Could you check a few things on this drawing? It's one solid part, dimensions in mm from its lowest x, y, z. Coordinates: 2 decimals unless noted, no trailing zeros. Write each loop counter-clockwise with the first axis right and the second up, starting at its lowest first coordinate (ties: lowest second). Pieces come first, ordered by that corner, then holes. Notation, with made-up numbers: M 13.5,-17 L 48.5,-17 A14 cw 48.5,2 Z; hole C 25.25,75 d1. An arc over 180 degrees is marked long. Use a Markdown table: item, result.
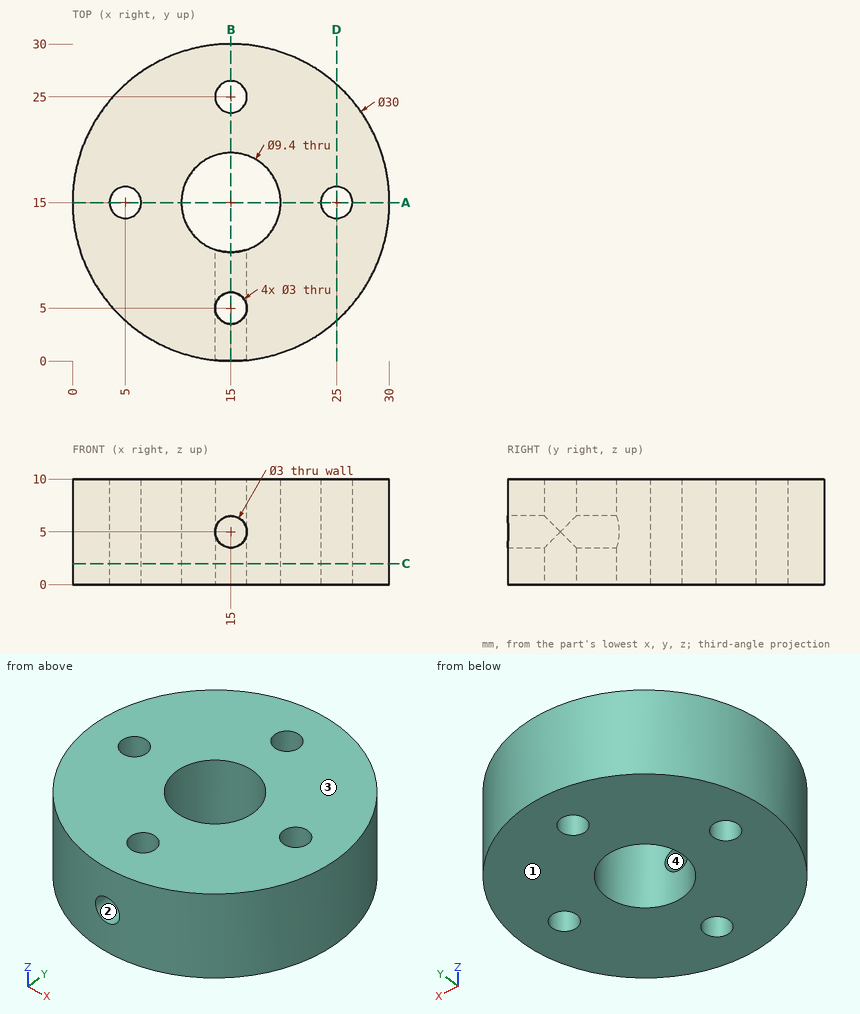
1. Suppose I cut it at C-C on z = 2. Write out the boundary of the cut face in (x, y), and give its area (3 significant figures).
Answers follow:
| item | result |
|---|---|
| outline | C 15,15 d30; hole C 5,15 d3; hole C 15,15 d9.4; hole C 15,5 d3; hole C 15,25 d3; hole C 25,15 d3 |
| area | 609 mm2 |
2. We'd pull the mould along Z, two halves only. Please class the marked faces 1, 2, 3 and 4: +Z half, -Z half, draft (parallel to the pull), parting line (faces both ways), or undercut.
Answers follow:
| item | result |
|---|---|
| face 1 | -Z half |
| face 2 | undercut |
| face 3 | +Z half |
| face 4 | undercut |
3. Will these pins go through, and if not, where does the flat tip stop? pin 1 Ø1.5 at (x, z) = (7, 4) entering from -Y; pin 2 Ø3 at (x, z) = (21.5, 2.5) entering from -Y; pin 3 Ø1.8 at (x, y) = (15, 25) entering from +Z; pin 4 Ø6 at (y, z) = (23.5, 6) entering from +X.
Answers follow:
| item | result |
|---|---|
| pin 1 | stops at y = 1.87 |
| pin 2 | stops at y = 0.86 |
| pin 3 | passes through |
| pin 4 | stops at x = 28.96 |
4. Suppose I cut it at D-D on x = 25. Write out the boundary of the cut face in (y, z), and give its area (3 significant figures).
Answers follow:
| item | result |
|---|---|
| outline | M 3.82,0 L 13.5,0 L 13.5,10 L 3.82,10 Z; M 16.5,0 L 26.18,0 L 26.18,10 L 16.5,10 Z |
| area | 194 mm2 |
5. I need wall thicknesses on probe 1 along Y at (x, z) = (15, 7.25); probe 2 along Y at (x, z) = (16, 2.5); probe 3 along Y at (x, z) = (5, 1.5). Which ranges of each line are inside material? Lowest first, please.
Answers follow:
| item | result |
|---|---|
| probe 1 | y = 0 to 3.5, 6.5 to 10.3, 19.7 to 23.5, 26.5 to 30 |
| probe 2 | y = 0.03 to 3.88, 6.12 to 10.41, 19.59 to 23.88, 26.12 to 29.97 |
| probe 3 | y = 3.82 to 13.5, 16.5 to 26.18 |
6. Suppose I cut it at B-B on x = 15. Write out the boundary of the cut face in (y, z), and give its area (3 significant figures).
Answers follow:
| item | result |
|---|---|
| outline | M 0,0 L 3.5,0 L 3.5,3.5 L 0,3.5 Z; M 0,6.5 L 3.5,6.5 L 3.5,10 L 0,10 Z; M 6.5,0 L 10.3,0 L 10.3,3.5 L 6.5,3.5 Z; M 6.5,6.5 L 10.3,6.5 L 10.3,10 L 6.5,10 Z; M 19.7,0 L 23.5,0 L 23.5,10 L 19.7,10 Z; M 26.5,0 L 30,0 L 30,10 L 26.5,10 Z |
| area | 124 mm2 |
7. Suppose I cut it at A-A on y = 15. Write out the boundary of the cut face in (x, z).
Answers follow:
| item | result |
|---|---|
| outline | M 0,0 L 3.5,0 L 3.5,10 L 0,10 Z; M 6.5,0 L 10.3,0 L 10.3,10 L 6.5,10 Z; M 19.7,0 L 23.5,0 L 23.5,10 L 19.7,10 Z; M 26.5,0 L 30,0 L 30,10 L 26.5,10 Z |
